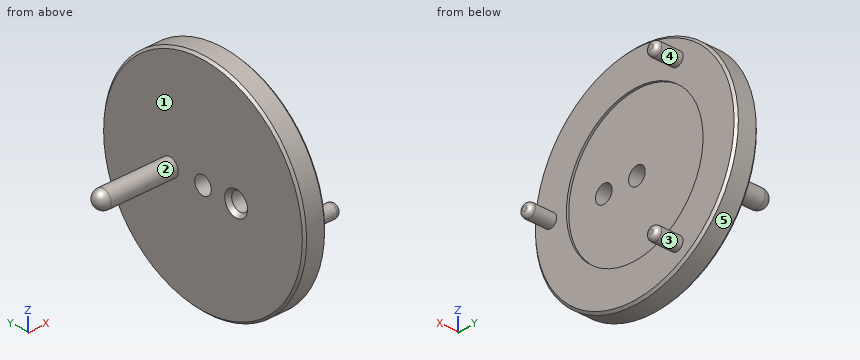
Autodesk Inventor part; units mm, degrees
ref_plane "YZ Plane" through (0, 0, 0) normal (1, 0, 0) x (0, 1, 0)
ref_plane "XZ Plane" through (0, 0, 0) normal (0, 1, 0) x (-1, 0, 0)
ref_plane "XY Plane" through (0, 0, 0) normal (0, 0, 1) x (1, 0, 0)
sketch "Sketch1" plane through (0, 0, 0) normal (1, 0, 0) x (0, 1, 0)
  circle A0 centre (0, 0) radius 38.8938
  dimension "d0" = 77.7875
extrude "Extrusion1" add sketch "Sketch1" along normal blind 7.9375
chamfer "Chamfer1" distance 0.7874 angle 45 2 edges at (7.9375, -38.8938, 0) (0, -38.8938, 0)
sketch "Sketch2" plane through (7.9375, 0, 0) normal (1, 0, 0) x (0, 0, -1)
  circle A0 centre (0, 0) radius 3.175
  dimension "d6" = 6.35
extrude "Extrusion2" cut sketch "Sketch2" against normal blind 7.9375
sketch "Sketch3" plane through (0, 0, 0) normal (-1, 0, 0) x (0, 0, 1)
  line L0 (0, 0) -> (0, -12.7)
  dimension "d9" = 12.7
hole "Hole1" at (0, -12.7, 0) direction (1, 0, 0) diameter 6.35 end through all countersink diameter 8.7376 countersink angle 82
sketch "Sketch4" plane through (0, 0, 0) normal (-1, 0, 0) x (0, 0, 1)
  point P0 (0, 0)
sketch "Sketch5" plane through (7.9375, 0, 0) normal (1, 0, 0) x (0, 0, -1)
  circle A0 centre (0, 0) radius 26.1938
  dimension "d17" = 52.3875
extrude "Extrusion3" cut sketch "Sketch5" against normal blind 0.7874
sketch "Sketch6" plane through (0, 0, 0) normal (-1, 0, 0) x (0, 0, 1)
  line L0 (0, 0) -> (0, 12.7)
  circle A0 centre (0, 12.7) radius 3.175
  dimension "d20" = 12.7
  dimension "d21" = 6.35
extrude "Extrusion4" add sketch "Sketch6" along normal blind 22.225
sketch "Sketch7" plane through (-22.225, 12.7, 0) normal (-1, 0, 0) x (0, 0, 1)
  circle A0 centre (0, 0) radius 3.175
  circle A1 centre (0, 0) radius 3.175
  point P0 (0, -12.7)
extrude "Extrusion5" add sketch "Sketch7" along normal blind 4.7625
fillet "Fillet1" radius 3.175 1 edges at (-26.9875, 12.7, -3.175)
sketch "Sketch8" plane through (7.9375, 0, 0) normal (1, 0, 0) x (0, 0, -1)
  circle A0 centre (0, -32.3239) radius 2.3813
  circle A1 centre (27.9933, 16.162) radius 2.3813
  circle A2 centre (-27.9933, 16.162) radius 2.3813
  point P0 (0, 0)
  dimension "d27" = 4.7625
  dimension "d30" = 360
extrude "Extrusion6" add sketch "Sketch8" along normal blind 4.7625
sketch "Sketch9" plane through (12.7, 16.162, -27.9933) normal (1, 0, 0) x (0, 0, -1)
  circle A0 centre (0, 0) radius 2.3813
  point P0 (-27.9933, -16.162)
extrude "Extrusion7" add sketch "Sketch9" along normal blind 4.445
fillet "Fillet2" radius 1.5875 1 edges at (17.145, 16.162, -25.6121)
sketch "Sketch10" plane through (12.7, 16.162, 27.9933) normal (1, 0, 0) x (0, 0, -1)
  circle A0 centre (0, 0) radius 2.3813
  circle A1 centre (0, 0) radius 2.3813
  point P0 (27.9933, -16.162)
extrude "Extrusion8" add sketch "Sketch10" along normal blind 4.445
fillet "Fillet3" radius 1.5875 1 edges at (17.145, 16.162, 30.3746)
sketch "Sketch11" plane through (12.7, -32.3239, 0) normal (1, 0, 0) x (0, 0, -1)
  circle A0 centre (0, 0) radius 2.3813
  circle A1 centre (0, 0) radius 2.3813
  point P0 (0, 32.3239)
extrude "Extrusion9" add sketch "Sketch11" along normal blind 4.445
fillet "Fillet4" radius 1.5875 1 edges at (17.145, -32.3239, 2.3813)
properties part number "idk"
Geometry: final body of the model. Coordinates: model frame, mm. Face numbers are marked on the shaded views. A direction names the side the tool comes from. Coordinates: 2 decimals unless noted, no trailing zeros. Order: outer loops, then holes, each group sorted by start corner. A loop starts at its lowest first (then second) coordinate and runs counter-clockwise, first axis right, second up.
Item 1: Section query B-B (x = 2.5). Output: boundary loops of the cut face in (y, z) (3 decimals), then the cut area to 3 significant figures.
Answer:
outline: circle Ø77.788 at (0, 0); hole circle Ø6.35 at (-12.7, 0); hole circle Ø6.35 at (0, 0)
area: 4,690 mm2
Item 2: Access query for the marked faces 4 and 5. Directions: +Z, -Z, +X, -X, +Y, -Y. A direction counts if a zero-diameter tool reaches every point of the face in a straight line with its end or side. Return the directions, or none.
Answer:
face 4: +X
face 5: +X, -X
Item 3: Section query D-D (x = -10.5). Output: boundary loops of the cut face in (y, z) (3 decimals).
Answer:
outline: circle Ø6.35 at (12.7, 0)
Item 4: Contact query for flat-ended pins moving along their axis: P1, Ø6, axis at x = -1, z = -14, coming from the -Y side; P2, Ø1, axis at y = 16, z = 15, coming from the -X side; P3, Ø2, axis at x = 4.5, z = -17, coming from the -Y side. Output: stop coordinate, or through.
Answer:
P1: stops at y = -37.13
P2: stops at x = 0
P3: stops at y = -35.45
Item 5: Section query A-A (y = 0). Output: boundary loops of the cut face in (x, z) (1 decimal), then the cut area to 3 significant figures.
Answer:
outline: (0, -38.1) - (0.8, -38.9) - (7.2, -38.9) - (7.9, -38.1) - (7.9, -26.2) - (7.2, -26.2) - (7.2, -3.2) - (0, -3.2) - close; (0, 3.2) - (7.2, 3.2) - (7.2, 26.2) - (7.9, 26.2) - (7.9, 38.1) - (7.2, 38.9) - (0.8, 38.9) - (0, 38.1) - close
area: 530 mm2
Item 6: Draft query along Z for the marked faces 1, 2 and 3. Return one class per face: released by +Z, released by -Z, zero draft, split by the parting line, or undercut.
Answer:
face 1: zero draft
face 2: split by the parting line
face 3: undercut
Item 7: Material intervals for line 1 along X through (y, z) = (-19.5, -18); line 2 along X through (y, z) = (5, 16.5); line 3 along Z through (x, y) = (2, -12), sorted ascending.
Answer:
line 1: x = 0 to 7.94
line 2: x = 0 to 7.15
line 3: z = -37 to -3.1, 3.1 to 37
Item 8: Section query C-C (x = 10.5). Output: boundary loops of the cut face in (y, z).
Answer:
outline: circle Ø4.76 at (-32.32, 0); circle Ø4.76 at (16.16, -27.99); circle Ø4.76 at (16.16, 27.99)
